Source: CAD feature listing. Evaluate the final solid. Frame: model axes, mm. A direction names the side the tool comes from. Give positions to 0.01 mm unless a question says otherwise; leave off trailing zeros. Write each loop counter-clockwise with the first axis right and the second up, starting at its lowest first coordinate (ties: lowest second). Pieces come first, ordered by that corner, then holes. Notation, with made-up numbers: (-21.75, -16.5) - (-7.75, -16.5) arc R30 ccw to (-7.75, 10.5) - close; hole circle Ø11 at (64, 71.5). An arc over 180 degrees is marked (long way). Answer as a JSON object with one key per item and string values. Group by question number.
from build123d import *

# Parameters (mm, degrees)
SKETCH2_R          = 1
CUT_EXTRUDE1_DEPTH = 4
SKETCH3_R          = 1
CUT_EXTRUDE2_DEPTH = 3


with BuildPart() as part:
    # Sketch1 → Revolve1 (revolve)
    with BuildSketch(Plane.XY):
        Polygon((0, 21.642718579), (0, 0), (0, -2.157281421), (1, -2.157281421), (1, -0.357281421), (10.085786438, -0.357281421), (11.5, 1.056932142), (11.5, 2.056932142), (11, 2.056932142), (11, 2.556932142), (11.5, 2.556932142), (11.5, 3.556932142), (9.5, 3.556932142), (9.5, 3.856932142), (11.5, 3.856932142), (11.5, 15.314291455), (8.671572875, 18.142718579), (1, 18.142718579), (1, 21.642718579), align=None)
        Polygon((2, 17.142718579), (8.257359313, 17.142718579), (10.5, 14.900077892), (10.5, 10.467720713), (1, 10.467720713), (1, 16.142718579), (2, 16.142718579), align=None, mode=Mode.SUBTRACT)
    revolve(axis=Axis((0, 21.642718579, 0), (0, -1, 0)))

    # Sketch2 → Cut-Extrude1 (cut)
    with BuildSketch(Plane(origin=(0, 18.142718579, 0), x_dir=(1, 0, 0), z_dir=(0, 1, 0))):
        with Locations((0, -4.5)):
            Circle(SKETCH2_R)
        with Locations((-4.5, 0)):
            Circle(SKETCH2_R)
        with Locations((0, 4.5)):
            Circle(SKETCH2_R)
        with Locations((4.5, 0)):
            Circle(SKETCH2_R)
        with BuildLine():
            Line((-3, 9.824499933), (-3, 15.547294435))
            Line((-3, 15.547294435), (3, 15.547294435))
            Line((3, 15.547294435), (3, 9.824499933))
            ThreePointArc((3, 9.824499933), (0, 6.824499933), (-3, 9.824499933))
        make_face()
        with BuildLine():
            Line((11.964351941, 10.371723429), (14.964351941, 5.175571006))
            Line((14.964351941, 5.175571006), (10.008266522, 2.314173755))
            ThreePointArc((10.008266522, 2.314173755), (5.91019031, 3.412249967), (7.008266522, 7.510326178))
            Line((7.008266522, 7.510326178), (11.964351941, 10.371723429))
        make_face()
        with BuildLine():
            Line((14.964351941, -5.175571006), (11.964351941, -10.371723429))
            Line((11.964351941, -10.371723429), (7.008266522, -7.510326178))
            ThreePointArc((7.008266522, -7.510326178), (5.91019031, -3.412249967), (10.008266522, -2.314173755))
            Line((10.008266522, -2.314173755), (14.964351941, -5.175571006))
        make_face()
        with BuildLine():
            Line((3, -15.547294435), (-3, -15.547294435))
            Line((-3, -15.547294435), (-3, -9.824499933))
            ThreePointArc((-3, -9.824499933), (0, -6.824499933), (3, -9.824499933))
            Line((3, -9.824499933), (3, -15.547294435))
        make_face()
        with BuildLine():
            Line((-11.964351941, -10.371723429), (-14.964351941, -5.175571006))
            Line((-14.964351941, -5.175571006), (-10.008266522, -2.314173755))
            ThreePointArc((-10.008266522, -2.314173755), (-5.91019031, -3.412249967), (-7.008266522, -7.510326178))
            Line((-7.008266522, -7.510326178), (-11.964351941, -10.371723429))
        make_face()
        with BuildLine():
            Line((-14.964351941, 5.175571006), (-11.964351941, 10.371723429))
            Line((-11.964351941, 10.371723429), (-7.008266522, 7.510326178))
            ThreePointArc((-7.008266522, 7.510326178), (-5.91019031, 3.412249967), (-10.008266522, 2.314173755))
            Line((-10.008266522, 2.314173755), (-14.964351941, 5.175571006))
        make_face()
    extrude(amount=-CUT_EXTRUDE1_DEPTH, mode=Mode.SUBTRACT)

    # Sketch3 → Cut-Extrude2 (cut)
    with BuildSketch(Plane.XZ.offset(0.357281421)):
        with Locations((0, -6)):
            Circle(SKETCH3_R)
        with Locations((0, 6)):
            Circle(SKETCH3_R)
        with Locations((-8, 0)):
            Circle(SKETCH3_R)
        with Locations((8, 0)):
            Circle(SKETCH3_R)
    extrude(amount=-CUT_EXTRUDE2_DEPTH, mode=Mode.SUBTRACT)


solid = part.part
Q1. Section B-B on z = -4.5. State how many separate pieces and enclosed holes the cut face has, then the cut area to 3 significant figures.
Q2. Section C-C on y = 4.5. Return the cut outline in (x, z).
Q3. Section A-A on y = 12.75. Return the cut outline in (x, z), then the cut area to 3 significant figures.
Q4. Reachability of faces 1 (the flat face through (3, 15.1, -10.5)), 2 (the cylindrical face through (-0.13, 17.65, -5.49)), 3 (the flat face through (7.569, 15.093, 7.834)), 4 (the conical face through (9.4, 16, 0)), 5 (the flat face through (-8, 2.643, 0)) from +Z, -Z, +X, -X, +Y, -Y: full face, straight path, thin tool, end or side. Return the list, or none.
Q5. First-contact query: pin 1 Ø1.6 at (x, z) = (-8, 0) entering from +Y; pin 2 Ø1.2 at (x, z) = (1.5, -10.5) entering from +Y; pin 3 Ø1.5 at (x, y) = (7, 9.5) entering from +Z. Flat tips, straight axial feed; report the tip coordinate or a pass-through.
Q6. Draft query along Z for faces 6 (the cylindrical face through (-1.5, 1.6, 11.4)), 7 (the conical face through (-5.001, 16.748, 8.736)), 8 (the flat face through (8, 2.643, 0)). Return one class per face: released by +Z, released by -Z, zero draft, split by the parting line, or undercut.
Q7. Ray query, probe 1 along Z at (x, y) = (0, 1.05); probe 2 along Y at (x, z) = (5.5, -4.5); probe 3 along Y at (x, z) = (7.75, 6.25). Return the intervals inside material, ascending. Write a range as [from, to].
Taken from the geometry:
{
 "1": {"separate pieces": "3", "enclosed holes": "0", "area": "242 mm²"},
 "2": {"outline": "circle Ø23 at (0, 0)"},
 "3": {"outline": "circle Ø23 at (0, 0); circle Ø2 at (0, 0); hole circle Ø21 at (0, 0)", "area": "72.3 mm²"},
 "4": {"face 1": "-Z, +Y", "face 2": "+Y", "face 3": "+X, +Y", "face 4": "none", "face 5": "-Y"},
 "5": {"pin 1": "stops at y = 18.14", "pin 2": "stops at y = 14.14", "pin 3": "stops at z = 9.65"},
 "6": {"face 6": "split by the parting line", "face 7": "released by +Z", "face 8": "undercut"},
 "7": {"probe 1": "z = [-11.49, -7], [-5, 5], [7, 11.49]", "probe 2": "y = [-0.36, 10.47], [17.14, 18.14]", "probe 3": "y = [-0.36, 3.56], [3.86, 10.47]"}
}
